For this review, take the finished solid that the model builds, in its own axes (mm). Give positions to 0.01 mm unless a question says otherwise; leave off trailing zeros. Write each loop counter-clockwise with the first axis right and the second up, starting at its lowest first coordinate (ties: lowest second). Pieces come first, ordered by that corner, then holes. Notation, with made-up numbers: (65.5, 67) -> (94.5, 67) arc R28 cw to (94.5, 106) -> close; hole circle Ø6 at (-38.5, 66.5). An arc over 180 degrees is marked (long way). Write item = value, one per line.
```python
from build123d import *

# Parameters (mm, degrees)
SKETCH_R   = 11
SKETCH_R_2 = 1.5
SKETCH_R_3 = 5
PAD_DEPTH  = 6


with BuildPart() as part:
    # Sketch → Pad (new body)
    with BuildSketch(Plane.XY):
        Circle(SKETCH_R)
        with Locations((0, 8)):
            Circle(SKETCH_R_2, mode=Mode.SUBTRACT)
        with Locations((-8, 0)):
            Circle(SKETCH_R_2, mode=Mode.SUBTRACT)
        with Locations((0, -8)):
            Circle(SKETCH_R_2, mode=Mode.SUBTRACT)
        with Locations((8, 0)):
            Circle(SKETCH_R_2, mode=Mode.SUBTRACT)
        Circle(SKETCH_R_3, mode=Mode.SUBTRACT)
    extrude(amount=PAD_DEPTH)


solid = part.part
```
(1) Take a section at C-C (z = 1.9). Write out the cut boundary in (x, y), plus the area to 3 significant figures.
Answers below:
outline = circle Ø22 at (0, 0); hole circle Ø3 at (-8, 0); hole circle Ø10 at (0, 0); hole circle Ø3 at (0, -8); hole circle Ø3 at (0, 8); hole circle Ø3 at (8, 0)
area = 273 mm^2
(2) Take a section at B-B (x = -7.75). Write out the cut boundary in (y, z), plus the area to 3 significant figures.
Answers below:
outline = (-7.81, 0) -> (-1.48, 0) -> (-1.48, 6) -> (-7.81, 6) -> close; (1.48, 0) -> (7.81, 0) -> (7.81, 6) -> (1.48, 6) -> close
area = 75.9 mm^2
(3) The part is to be moulded in two halves that separate along Y. For faces 1 (the face through (-2.38, -10.74, 2.96)), 2 (the face through (6.5, 0.07, 2.96)), 3 (the face through (-1.08, -4.88, 2.96)), 4 (the face through (5, -2, 0)), say which applies: released by +Y, released by -Y, zero draft, split by the parting line, or undercut.
Answers below:
face_1 = split by the parting line
face_2 = undercut
face_3 = undercut
face_4 = zero draft
(4) Take a section at D-D (y = -8). Write out the cut boundary in (x, z), plus the area to 3 significant figures.
Answers below:
outline = (-7.55, 0) -> (-1.5, 0) -> (-1.5, 6) -> (-7.55, 6) -> close; (1.5, 0) -> (7.55, 0) -> (7.55, 6) -> (1.5, 6) -> close
area = 72.6 mm^2
(5) To check wall thickness, follow probe 1 along Y at (x, z) = (0, 3.9); probe 2 along Y at (x, z) = (-0.5, 1.4); probe 3 along Y at (x, z) = (8, 1.9). State the ranges of each line that lie inside material, in increasing order.
Answers below:
probe_1 = -11 to -9.5, -6.5 to -5, 5 to 6.5, 9.5 to 11
probe_2 = -10.99 to -9.41, -6.59 to -4.97, 4.97 to 6.59, 9.41 to 10.99
probe_3 = -7.55 to -1.5, 1.5 to 7.55
(6) For pin 1 (2.5 mm diameter, centred on x = -8, y = 0, fed in from +Z); pin 2 (2 mm diameter, centred on x = 2, z = 3, fed in from +Y); pin 3 (3 mm diameter, centred on y = -5, z = 5, fed in from -X); pin 4 (2 mm diameter, centred on x = -8, z = 2.5, fed in from -Y), all flat-tipped, find the tip position at first contact; note any pin that passes through.
Answers below:
pin_1 = through
pin_2 = 10.95
pin_3 = -10.43
pin_4 = -8.49
(7) Take a section at A-A (y = 0). Write out the cut boundary in (x, z).
Answers below:
outline = (-11, 0) -> (-9.5, 0) -> (-9.5, 6) -> (-11, 6) -> close; (-6.5, 0) -> (-5, 0) -> (-5, 6) -> (-6.5, 6) -> close; (5, 0) -> (6.5, 0) -> (6.5, 6) -> (5, 6) -> close; (9.5, 0) -> (11, 0) -> (11, 6) -> (9.5, 6) -> close
